Can you work these out from the model? Positions are in its coordinate system, mm. Face numbers are marked on the shaded views. A direction names the side the tool comes from. Round coordinates to 2 decimals unless told otherwise and drop trailing zeros. Order: outer loops, then holes, each group sorted by start corner. A loop starts at its lowest first (then second) coordinate and runs counter-clockwise, first axis right, second up.
Q1. If we section it at A-A (x = -2): Please give me the cut outline in (y, z).
Q2. For the marked faces 5, 6 and 7, which set-ups out of +Z, -Z, +X, -X, +Y, -Y let a thin tool reach every point of the face, with its end or its side?
Q3. If we section it at C-C (z = 1.8): Please give me the cut outline in (x, y).
Q4. Will these pins go through, and if not, where does the flat tip stop? P1, Ø5, axis at x = 2, y = -2, coming from the -Z side; P2, Ø3, axis at x = 3.5, y = -7.5, coming from the +Z side; P3, Ø1, axis at x = -0.5, y = -7.5, coming from the -Z side.
Q5. If we section it at D-D (x = -3): Please give me the cut outline in (y, z).
Q6. We'd pull the mould along Z, two halves only. Please class the marked faces 1, 2, 3 and 4: pulls with the +Z half, pulls with the -Z half, needs draft (parallel to the pull), parting line crosses it, or undercut.
Q7. If I drill on line 1 (X direction, y = -5.5, z = 2.85); line 2 (Z direction, x = -4.5, y = -1); line 3 (Z direction, x = -2, y = -8.5), over which ranges is the centre line in solid material (lowest first)?
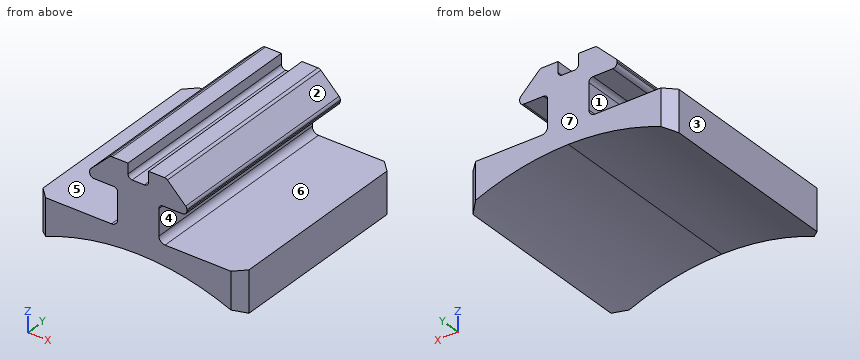
from build123d import *

# Parameters (mm, degrees)
F1_DEPTH = 10
F2_R     = 0.2
F3_R     = 0.3
F4_SIZE  = 0.5


# Not quite as in the source:
# - a feature names something its author has since deleted; it is built from what else it names


with BuildPart() as f1:
    # F0 (on Front) → F1 (new body)
    with BuildSketch(Plane.XZ):
        with BuildLine():
            Line((-5, 0.8663841993), (-5, -1.1336158007))
            ThreePointArc((-5, -1.1336158007), (-2.5588527336, -0.3183237919), (0, -0.0423279154))
            ThreePointArc((0, -0.0423279154), (2.5588527336, -0.3183237919), (5, -1.1336158007))
            Line((5, -1.1336158007), (5, 0.8663841993))
            Line((5, 0.8663841993), (1, 0.8663841993))
            Line((1, 0.8663841993), (1, 2.6280805469))
            Line((1, 2.6280805469), (2.3511576001, 2.6280805469))
            Line((2.3511576001, 2.6280805469), (2.363298554, 2.9764297366))
            Line((2.363298554, 2.9764297366), (1.357049332, 3.9621986704))
            Line((1.357049332, 3.9621986704), (0.5, 3.9621986704))
            Line((0.5, 3.9621986704), (0.5, 3.2621986704))
            Line((0.5, 3.2621986704), (0, 3.2621986704))
            Line((0, 3.2621986704), (-0.5, 3.2621986704))
            Line((-0.5, 3.2621986704), (-0.5, 3.9621986704))
            Line((-0.5, 3.9621986704), (-1.357049332, 3.9621986704))
            Line((-1.357049332, 3.9621986704), (-2.363298554, 2.9764297366))
            Line((-2.363298554, 2.9764297366), (-2.3511576001, 2.6280805469))
            Line((-2.3511576001, 2.6280805469), (-1, 2.6280805469))
            Line((-1, 2.6280805469), (-1, 0.8663841993))
            Line((-1, 0.8663841993), (-5, 0.8663841993))
        make_face()
    extrude(amount=F1_DEPTH)

    # F2
    f2_edges = [f1.edges().sort_by_distance(p)[0] for p in [
        (-0.5, -5, 3.262199),
        (0.5, -5, 3.262199),
        (2.351158, -5, 2.628081),
        (1, -5, 2.628081),
        (2.363299, -5, 2.97643),
        (1.357049, -5, 3.962199),
        (-1, -5, 2.628081),
        (-2.351158, -5, 2.628081),
        (-2.363299, -5, 2.97643),
        (-1.357049, -5, 3.962199),
    ]]
    fillet(f2_edges, radius=F2_R)

    # F3
    f3_edges = [f1.edges().sort_by_distance(p)[0] for p in [
        (-1, -5, 0.866384),
        (1, -5, 0.866384),
    ]]
    fillet(f3_edges, radius=F3_R)

    # F4
    f4_edges = [f1.edges().sort_by_distance(p)[0] for p in [
        (-5, -10, -0.133616),
        (5, -10, -0.133616),
        (5, 0, -0.133616),
        (-5, 0, -0.133616),
    ]]
    chamfer(f4_edges, length=F4_SIZE)


solid = f1.part
Solution:
1. outline: (-10, -0.21) - (0, -0.21) - (0, 0.87) - (-10, 0.87) - close; (-10, 2.63) - (0, 2.63) - (0, 3.33) - (-10, 3.33) - close
2. face 5: -X, +Y, -Y
2. face 6: +X, +Y, -Y
2. face 7: +Z, -Z, +X, -X, +Y
3. outline: (-1, -10) - (1, -10) - (1, 0) - (-1, 0) - close
4. P1: stops at z = -0.92
4. P2: stops at z = 3.33
4. P3: stops at z = -0.08
5. outline: (-10, -0.42) - (0, -0.42) - (0, 0.87) - (-10, 0.87) - close
6. face 1: undercut
6. face 2: pulls with the +Z half
6. face 3: needs draft
6. face 4: undercut
7. line 1: x = -2.36 to 2.36
7. line 2: z = -0.92 to 0.87
7. line 3: z = -0.21 to 0.87, 2.63 to 3.33
